Build history of the part. All positions in model axes, mm. Give positions to 0.01 mm unless a question says otherwise; leave off trailing zeros. Order: outer loops, then holes, each group sorted by start corner. A loop starts at its lowest first (then second) coordinate and runs counter-clockwise, first axis right, second up. Notation, with made-up numbers: (-10.75, -35.5) - (12.25, -35.5) arc R25 ccw to (12.25, -15.5) - close; hole circle Ø4 at (-8.5, -25). An arc over 180 degrees is marked (long way). Use a Markdown table: item, result. Add a question column.
(1) Slice it at D-D (z = 48). Write the cut outline in (x, y).
(2) Slice it at C-C (x = 29.5). Count the separate pieces of the cut face and the enclosed holes in it, then the cut area to 3 significant figures.
(3) Slice it at A-A (z = 29). Write the cut outline in (x, y).
(4) Mould opens along Y. For faces 1 (the face through (22.003, -79.036, 40.806)), 2 (the face through (10.2, -78.9, 40.8)), 3 (the face through (15, 0, 32)) say: +Y half, -Y half, draft (parallel to the pull), parting line (faces both ways), or undercut.
(5) Wall check: line 1 (Z direction, x = 28, y = -140.5); line 2 (X direction, y = -123, z = 31); line 3 (X direction, y = -133, z = 57.5) (3 decimals). Give the ranges that are in metal, low to high.
(6) Flat gauge pins, fed straight in: pin 1 (2 mm diameter, centred on y = -109.5, z = 71.5, fed in from -X) (3 decimals); pin 2 (3 mm diameter, centred on y = -30.5, z = 64.5, fed in from +X); pin 3 (6 mm diameter, centred on x = 25, y = -87.5, fed in from -Z). Where does each tip first touch, or does it go through?
(7) Slice it at B-B (x = 14.5). Write the cut outline in (y, z), then the cut area to 3 significant figures.
from build123d import *

# Parameters (mm, degrees)
PAD_DEPTH    = 160
SKETCH001_R  = 180
POCKET_DEPTH = 80.001
FILLET_R     = 10
CHAMFER_SIZE = 0.5


with BuildPart() as obj1:
    # Sphere002 → Sphere002 (revolve)
    with BuildSketch(Plane(origin=(31, -140, 10), x_dir=(1, 0, 0), z_dir=(0, -1, 0))):
        with BuildLine():
            ThreePointArc((0, -5), (5, 0), (0, 5))
            Line((0, 5), (0, -5))
        make_face()
    revolve(axis=Axis((31, -140, 10), (0, 0, 1)))


with BuildPart() as obj2:
    # Sphere003 → Sphere003 (revolve)
    with BuildSketch(Plane(origin=(31, -140, 70), x_dir=(1, 0, 0), z_dir=(0, -1, 0))):
        with BuildLine():
            ThreePointArc((0, -5), (5, 0), (0, 5))
            Line((0, 5), (0, -5))
        make_face()
    revolve(axis=Axis((31, -140, 70), (0, 0, 1)))


with BuildPart() as obj3:
    # Sphere001 → Sphere001 (revolve)
    with BuildSketch(Plane(origin=(31, -20, 70), x_dir=(1, 0, 0), z_dir=(0, -1, 0))):
        with BuildLine():
            ThreePointArc((0, -5), (5, 0), (0, 5))
            Line((0, 5), (0, -5))
        make_face()
    revolve(axis=Axis((31, -20, 70), (0, 0, 1)))


with BuildPart() as obj4:
    # Sphere → Sphere (revolve)
    with BuildSketch(Plane(origin=(31, -20, 10), x_dir=(1, 0, 0), z_dir=(0, -1, 0))):
        with BuildLine():
            ThreePointArc((0, -5), (5, 0), (0, 5))
            Line((0, 5), (0, -5))
        make_face()
    revolve(axis=Axis((31, -20, 10), (0, 0, 1)))


with BuildPart() as chamfer_body:
    # Sketch → Pad (new body)
    with BuildSketch(Plane.XZ):
        Polygon((0, 0), (35, 0), (35, 80), (20, 80), align=None)
    extrude(amount=PAD_DEPTH)

    # Sketch001 → Pocket (cut, through all)
    with BuildSketch(Plane(origin=(0, 0, 80), x_dir=(-1, 0, 0), z_dir=(0, 0, 1))):
        with Locations((-202, 80)):
            Circle(SKETCH001_R)
    extrude(amount=-POCKET_DEPTH, mode=Mode.SUBTRACT)

    # Fillet
    fillet_edges = [chamfer_body.edges().sort_by_distance(p)[0] for p in [
        (35, 0, 40),
        (35, -160, 40),
    ]]
    fillet(fillet_edges, radius=FILLET_R)

    # Cut: cut obj4
    add(obj4.part, mode=Mode.SUBTRACT)

    # Cut001: cut obj3
    add(obj3.part, mode=Mode.SUBTRACT)

    # Cut002: cut obj2
    add(obj2.part, mode=Mode.SUBTRACT)

    # Cut003: cut obj1
    add(obj1.part, mode=Mode.SUBTRACT)

    # Chamfer
    chamfer_edges = [chamfer_body.edges().sort_by_distance(p)[0] for p in [
        (12.5, 0, 0),
        (32.071068, -2.928932, 0),
        (0, -80, 0),
        (35, -11.418011, 0),
        (12.5, -160, 0),
        (25.279882, -45.794737, 0),
        (32.071068, -157.071068, 0),
        (25.279882, -114.205263, 0),
        (35, -148.581989, 0),
    ]]
    chamfer(chamfer_edges, length=CHAMFER_SIZE)


solid = chamfer_body.part
Solution:
| question | item | result |
|---|---|---|
| 1 | outline | (12, -160) - (25, -160) arc R10 ccw to (35, -150) - (35, -147.16) arc R180 cw to (35, -12.84) - (35, -10) arc R10 ccw to (25, 0) - (12, 0) - close |
| 2 | separate pieces | 2 |
| 2 | enclosed holes | 4 |
| 2 | area | 4,120 mm2 |
| 3 | outline | (7.25, -160) - (25, -160) arc R10 ccw to (35, -150) - (35, -147.16) arc R180 cw to (35, -12.84) - (35, -10) arc R10 ccw to (25, 0) - (7.25, 0) - close |
| 4 | face 1 | undercut |
| 4 | face 2 | draft |
| 4 | face 3 | +Y half |
| 5 | line 1 | 0 to 6.03, 13.97 to 66.03, 73.97 to 80 |
| 5 | line 2 | 7.75 to 27.21 |
| 5 | line 3 | 14.375 to 29.98 |
| 6 | pin 1 | x = 17.625 |
| 6 | pin 2 | x = 29.38 |
| 6 | pin 3 | z = 0.34 |
| 7 | outline | (-160, 0.5) - (-159.5, 0) - (-0.5, 0) - (0, 0.5) - (0, 58) - (-160, 58) - close |
| 7 | area | 9,280 mm2 |
